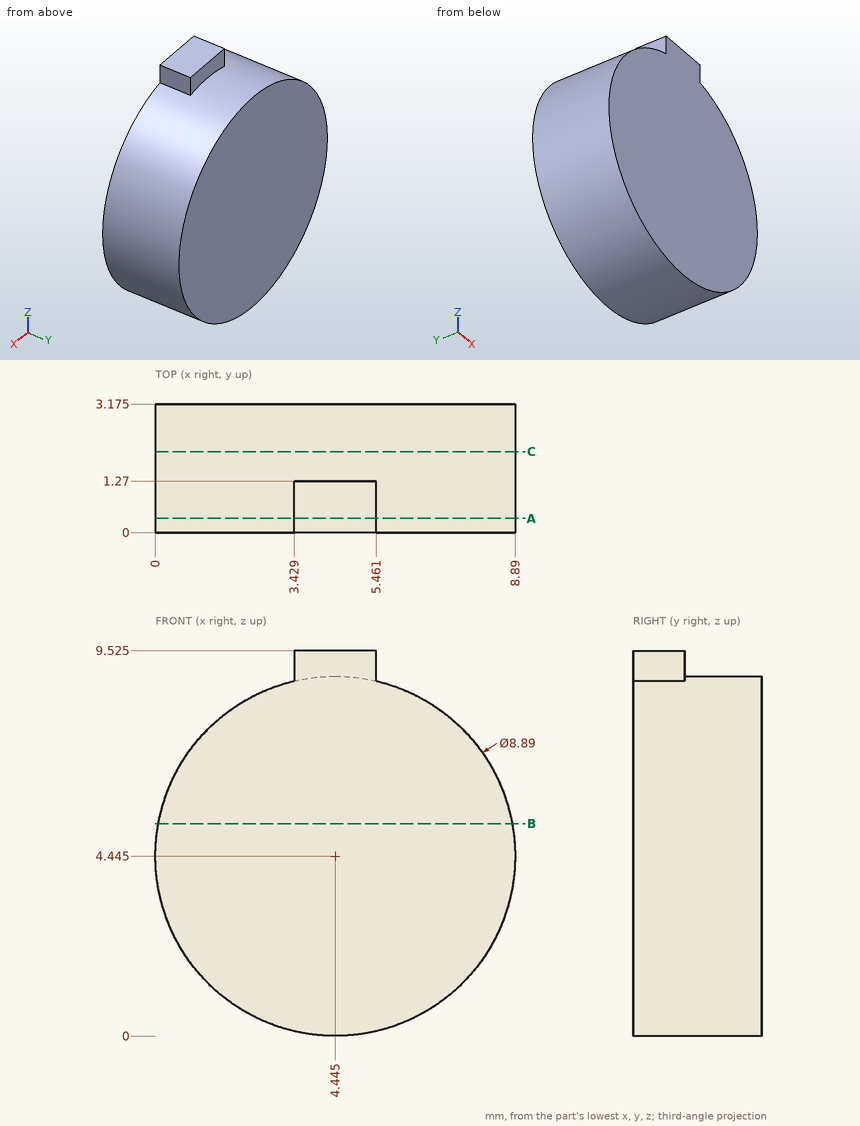
Drawing for the job (mm, zero at the part's lowest x, y, z). Coordinates: 2 decimals unless noted, no trailing zeros. Loops run counter-clockwise (first coordinate to the right, second up) from the corner with the lowest first, then second, coordinate; pieces in that order, holes last. Notation, with made-up numbers: (43.25, -39) - (57.25, -39) arc R28 ccw to (57.25, -7) - close; hole circle Ø11 at (57.5, -16). An arc over 180 degrees is marked (long way). Use CSV: the item, a comma, the result in double quotes. Start each with the question number.
Q1. Probe probe 1 along Z at (x, y) = (2.5, 2.2); probe 2 along Z at (x, y) = (4.5, 1.85); probe 3 along X at (y, z) = (2.3, 7.75). List the from-to ranges inside material, lowest first. Write a range as from..to.
Q2. Cut at B-B, the plane z = 5.25. List the corners of the cut face in (x, y) (1 decimal), then the cut area to 3 significant figures.
Q3. Cut at C-C, the plane y = 2. List the corners of the cut face in (x, z) (3 decimals), then the cut area to 3 significant figures.
Q4. Cut at A-A, the plane y = 0.35. List the corners of the cut face in (x, z) (3 decimals), then the cut area to 3 significant figures.
Here are the results:
1,probe 1,"0.45..8.44"
1,probe 2,"0..8.89"
1,probe 3,"1.47..7.42"
2,outline,"(0.1, 0) - (8.8, 0) - (8.8, 3.2) - (0.1, 3.2) - close"
2,area,"27.8 mm2"
3,outline,"circle Ø8.89 at (4.445, 4.445)"
3,area,"62.1 mm2"
4,outline,"(3.429, 8.772) arc R4.445 ccw (long way) to (5.461, 8.772) - (5.461, 9.525) - (3.429, 9.525) - close"
4,area,"63.4 mm2"
